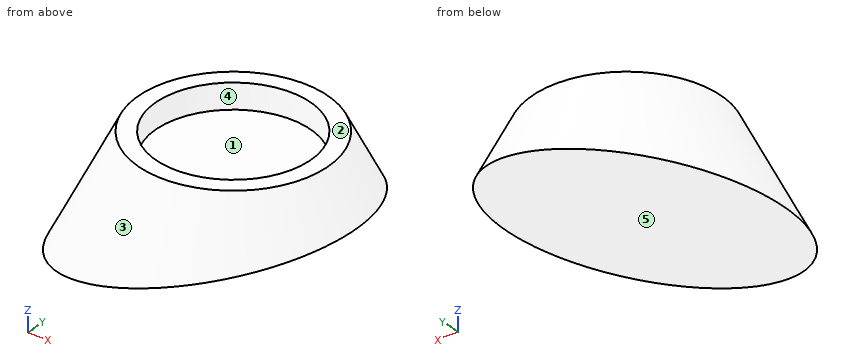
```python
from build123d import *

# Parameters (mm, degrees)
F0_R     = 12.5
F1_DEPTH = 10
F2_SIZE2 = 9.99999
F2_SIZE  = 4.99999
F4_DEPTH = 12.5
F5_R     = 6.125
F6_DEPTH = 2


# Not quite as in the source:
# - a fillet or chamfer is up to 0.001 mm smaller than in the source, because OpenCascade refuses the exact size


with BuildPart() as f1:
    # F0 (on Top) → F1 (new body)
    with BuildSketch(Plane.XY):
        Circle(F0_R)
    extrude(amount=F1_DEPTH)

    # F2 (size 5 and 10 in the source; OpenCascade refuses exactly that, so slightly less here)
    f2_edges = [f1.edges().sort_by_distance(p)[0] for p in [
        (-12.5, 0, 10),
    ]]
    f2_side = f1.faces().sort_by_distance((0, 0, 10))[0]
    chamfer(f2_edges, length=F2_SIZE, length2=F2_SIZE2, reference=f2_side)

    # F3 (on Front) → F4 (cut, symmetric)
    with BuildSketch(Plane.XZ):
        Polygon((11.7184263772, 6.5591478468), (-12.7606466413, 0), (-7.277042605, -3.8485343102), (16.1768086255, -2.4198731408), align=None)
    extrude(amount=F4_DEPTH, both=True, mode=Mode.SUBTRACT)

    # F5 (on face) → F6 (cut)
    with BuildSketch(Plane.XY.offset(10)):
        Circle(F5_R)
    extrude(amount=-F6_DEPTH, mode=Mode.SUBTRACT)


solid = f1.part
```
CAD build for the part. Positions are in the model's coordinates, mm. Face numbers are marked on the shaded views. A direction names the side the tool comes from. Round coordinates to 2 decimals unless told otherwise and drop trailing zeros. Order: outer loops, then holes, each group sorted by start corner. A loop starts at its lowest first (then second) coordinate and runs counter-clockwise, first axis right, second up.
Q1. Which spindle directions (+Z, -Z, +X, -X, +Y, -Y) get a long thin tool onto all of the face, cutting with end or side? Do the marked faces 1 and 2. Say none if no direction does.
Q2. Slice it at D-D (z = 6.5). Write the cut outline in (x, y).
Q3. Wall check: L1, parallel to Y at x = 0, z = 9.1 (3 decimals); L2, parallel to Y at x = 0, z = 8.9 (3 decimals); L3, parallel to Y at x = -6.25, z = 7.5. Give the ranges that are in metal, low to high.
Q4. Slice it at C-C (x = 0). Write the cut outline in (y, z) (3 decimals), and give its area (3 significant figures).
Q5. Drop flat-ended pins along their axis: pin 1 (1 mm diameter, centred on y = 6.5, z = 5, fed in from -X); pin 2 (1.5 mm diameter, centred on y = -2.5, z = 8, fed in from -X); pin 3 (1 mm diameter, centred on y = -8.5, z = 5.5, fed in from -X). Give the stop position or say it passes through.
Q6. Slice it at A-A (y = 0). Write the cut outline in (x, z) (3 decimals), and give its area (3 significant figures).
Q7. Two-plate mould, pull along Y, no slides. Class the marked faces 3, 4 and 5: pulls with the +Y half, pulls with the -Y half, needs draft (parallel to the pull), parting line crosses it, or undercut.
Q8. Slice it at B-B (z = 8.5). Write the cut outline in (x, y) (3 decimals), and give its area (3 significant figures).
Results below:
1. face 1: +Z
1. face 2: +Z, +X, -X, +Y, -Y
2. outline: circle Ø18.5 at (0, 0)
3. L1: y = -7.95 to -6.125, 6.125 to 7.95
3. L2: y = -8.05 to -6.125, 6.125 to 8.05
3. L3: y = -6.12 to 6.12
4. outline: (-10.79, 3.419) - (10.79, 3.419) - (7.5, 10) - (6.125, 10) - (6.125, 8) - (-6.125, 8) - (-6.125, 10) - (-7.5, 10) - close
4. area: 95.9 mm2
5. pin 1: stops at x = -8.11
5. pin 2: stops at x = -8.57
5. pin 3: stops at x = -5.7
6. outline: (-12.46, 0.081) - (9.516, 5.969) - (7.5, 10) - (6.125, 10) - (6.125, 8) - (-6.125, 8) - (-6.125, 10) - (-7.5, 10) - close
6. area: 100 mm2
7. face 3: parting line crosses it
7. face 4: undercut
7. face 5: needs draft
8. outline: circle Ø16.5 at (0, 0); hole circle Ø12.25 at (0, 0)
8. area: 96.0 mm2
